Input: part model. Units: mm. Frame: model coordinates. A direction names the side the tool comes from. Coordinates: 2 decimals unless noted, no trailing zeros. Loops run counter-clockwise (first coordinate to the right, second up) from the corner with the lowest first, then second, coordinate; pieces in that order, holes last.
(1) Set-up query: faces 1 (the face through (0, -12, -130)), 2 (the face through (142, -12, -12.5)), 3 (the face through (-117, -12, 12.5)), 4 (the face through (25, -12, 133)). Return all of +Z, -Z, +X, -X, +Y, -Y with unobstructed straight access to the full face (end or side cutting, diameter ignored); none if empty.
(2) Contact query for flat-ended pins moving along their axis: P1, Ø1.5, axis at y = -5, z = -104, coming from the +X side; P2, Ø12, axis at x = -20, y = -16.5, coming from the -Z side; P3, Ø10, axis at y = -10, z = -185, coming from the -X side. Output: stop coordinate, or through.
(3) Section C-C, the plane x = 84.5. Return loops of the section in (y, z).
(4) Section A-A, the plane y = -5.5. Return loops of the section in (x, z), then the cut area to 3 significant figures.
(5) Section B-B, the plane z = -52. Return loops of the section in (x, y).
(6) Line query: L1, parallel to X at y = -3.5, z = 100.5; L2, parallel to Z at x = 80, y = -8. Output: solid intervals per line, ascending.
```python
from build123d import *

# Parameters (mm, degrees)
F0_W     = 25
F0_H     = 250
F1_DEPTH = 25
F3_COUNT = 4


with BuildPart() as f1:
    # F0 (on Front) → F1 (new body)
    with BuildSketch(Plane.XZ):
        with Locations((12.5, 125)):
            Rectangle(F0_W, F0_H)
    extrude(amount=F1_DEPTH)


with BuildPart() as f3_1:
    # F3: instance of F1
    add(f1.part.rotate(Axis((12.5, -12.5, 0), (0, -1, 0)), 1 * 360 / F3_COUNT))


with BuildPart() as f3_2:
    # F3: instance of F1
    add(f1.part.rotate(Axis((12.5, -12.5, 0), (0, -1, 0)), 2 * 360 / F3_COUNT))


with BuildPart() as f3_3:
    # F3: instance of F1
    add(f1.part.rotate(Axis((12.5, -12.5, 0), (0, -1, 0)), 3 * 360 / F3_COUNT))


with BuildPart() as f3_2_1:
    add(f3_2.part)

    # F4: union F3_1, F1, F3_3
    add(f3_1.part)
    add(f1.part)
    add(f3_3.part)


solid = f3_2_1.part
```
Report:
1. face 1: -Z, -X, +Y, -Y
1. face 2: -Z, +X, +Y, -Y
1. face 3: +Z, -X, +Y, -Y
1. face 4: +Z, +X, +Y, -Y
2. P1: stops at x = 25
2. P2: stops at z = -12.5
2. P3: stops at x = 0
3. outline: (-25, -12.5) - (0, -12.5) - (0, 12.5) - (-25, 12.5) - close
4. outline: (-237.5, -12.5) - (0, -12.5) - (0, -250) - (25, -250) - (25, -12.5) - (262.5, -12.5) - (262.5, 12.5) - (25, 12.5) - (25, 250) - (0, 250) - (0, 12.5) - (-237.5, 12.5) - close
4. area: 24,400 mm2
5. outline: (0, -25) - (25, -25) - (25, 0) - (0, 0) - close
6. L1: x = 0 to 25
6. L2: z = -12.5 to 12.5
